```python
from build123d import *

# Parameters (mm, degrees)
ESBO_O1_R                = 1.5
RESSALTO_EXTRUS_O1_DEPTH = 2.4


with BuildPart() as part:
    # Esboço1 → Ressalto-extrusão1 (new body)
    with BuildSketch(Plane(origin=(0, 0, 0), x_dir=(1, 0, 0), z_dir=(0, 1, 0))):
        Polygon((3.175426481, 0), (1.58771324, 2.75), (-1.58771324, 2.75), (-3.175426481, 0), (-1.58771324, -2.75), (1.58771324, -2.75), align=None)
        Circle(ESBO_O1_R, mode=Mode.SUBTRACT)
    extrude(amount=RESSALTO_EXTRUS_O1_DEPTH)

    # Esboço3 → Corte-Revolução1 (revolve, cut)
    with BuildSketch(Plane.XY):
        with BuildLine():
            Line((1.5, 2.45), (1.5, 3.039454742))
            Line((1.5, 3.039454742), (3.5, 3.039454742))
            Line((3.5, 3.039454742), (3.5, 2.097346039))
            ThreePointArc((3.5, 2.097346039), (2.515426612, 2.361161683), (1.5, 2.45))
        make_face()
        with BuildLine():
            ThreePointArc((1.5, -0.05), (2.515426612, 0.038838317), (3.5, 0.302653961))
            Line((3.5, 0.302653961), (3.5, -0.837086604))
            Line((3.5, -0.837086604), (1.5, -0.837086604))
            Line((1.5, -0.837086604), (1.5, -0.05))
        make_face()
    revolve(axis=Axis((0, 0, 0), (0, 1, 0)), mode=Mode.SUBTRACT)


solid = part.part
```
The listing builds one solid part. Answer for the finished solid, in the listing's coordinates (mm). Give positions to 0.01 mm unless a question says otherwise; leave off trailing zeros. Order: outer loops, then holes, each group sorted by start corner. A loop starts at its lowest first (then second) coordinate and runs counter-clockwise, first axis right, second up.
Item 1: For a pull along X with two mould halves and no side action, classify faces 1 (the face through (-1.5, 1.18, -0.07)), 2 (the face through (-2.37, 1.184, -1.394)), 3 (the face through (0, 0, 2)) as pulls with the +X half, pulls with the -X half, needs draft (parallel to the pull), parting line crosses it, or undercut.
From the geometry:
face 1: undercut
face 2: pulls with the -X half
face 3: needs draft
Item 2: Find the intervals of material crossed by probe 1 along Z at (x, y) = (0, 0.8); probe 2 along X at (y, z) = (0.7, -1); probe 3 along Z at (x, y) = (0.5, 0.55), in increasing order.
From the geometry:
probe 1: z = -2.75 to -1.5, 1.5 to 2.75
probe 2: x = -2.6 to -1.12, 1.12 to 2.6
probe 3: z = -2.75 to -1.41, 1.41 to 2.75
Item 3: The part is cut by section A-A, the plane y = 1.2. Give the vertices of the cut face in (x, z), and give its area (3 significant figures).
From the geometry:
outline: (-3.18, 0) - (-1.59, -2.75) - (1.59, -2.75) - (3.18, 0) - (1.59, 2.75) - (-1.59, 2.75) - close; hole circle Ø3 at (0, 0)
area: 19.1 mm2
